from build123d import *

# Parameters (mm, degrees)
SKETCH_1_W        = 50
SKETCH_1_H        = 2
EXTRUDE_1_DEPTH   = 15
EXTRUDE_1_2_DEPTH = 15
SKETCH_2_W        = 50
SKETCH_2_H        = 12.8
EXTRUDE_2_DEPTH   = 2
FILLET_1_R        = 2


with BuildPart() as part:
    # Sketch 1 → Extrude 1 (new body)
    with BuildSketch(Plane.XY):
        with Locations((25, -1)):
            Rectangle(SKETCH_1_W, SKETCH_1_H)
    extrude(amount=EXTRUDE_1_DEPTH)



with BuildPart() as body_2:
    # Sketch 1 → Extrude 1 2 (new body)
    with BuildSketch(Plane.XY):
        with Locations((25, 9.8)):
            Rectangle(SKETCH_1_W, SKETCH_1_H)
    extrude(amount=EXTRUDE_1_2_DEPTH)


with BuildPart() as part_1:
    add(part.part)

    add(body_2.part)  # Extrude 2 merges body 2
    # Sketch 2 → Extrude 2 (add)
    with BuildSketch(Plane.XY.offset(15)):
        with Locations((25, 4.4)):
            Rectangle(SKETCH_2_W, SKETCH_2_H)
    extrude(amount=-EXTRUDE_2_DEPTH)

    # Fillet 1
    fillet_1_edges = [part_1.edges().sort_by_distance(p)[0] for p in [
        (25, 0, 0),
        (25, 8.8, 0),
    ]]
    fillet(fillet_1_edges, radius=FILLET_1_R - 0.0001)  # a hair under: the kernel refuses the full size


solid = part_1.part
Input: part model. Units: mm. Frame: model coordinates. A direction names the side the tool comes from. Give positions to 0.01 mm unless a question says otherwise; leave off trailing zeros. Order: outer loops, then holes, each group sorted by start corner. A loop starts at its lowest first (then second) coordinate and runs counter-clockwise, first axis right, second up. Notation, with made-up numbers: (78, -25.5) - (93, -25.5) arc R30 ccw to (93, 4.5) - close; hole circle Ø4 at (36, 77). An arc over 180 degrees is marked (long way). Answer as a JSON object with one key per item and string values. Group by question number.
Q1. First-contact query: pin 1 Ø2.5 at (x, y) = (37.5, 6.5) entering from -Z. Flat tip, straight axial feed; report the tip coordinate or a pass-through.
Q2. Cut plane C-C, the plane y = 6. Output: boundary loops of the cut face in (x, z).
Q3. Cut plane D-D, the plane y = 9.75. Output: boundary loops of the cut face in (x, z), then the cut area to 3 significant figures.
Q4. Line query: probe 1 along Y at (x, z) = (12, 2.25); probe 2 along Z at (x, y) = (25, 5.5); probe 3 along Y at (x, z) = (21, 1.5). Output: solid intervals per line, ascending.
Q5. Cut plane A-A, the plane z = 6.5. Output: boundary loops of the cut face in (x, y), then the cut area to 3 significant figures.
Q6. Mould query, pull axis Y, two halves, no side actions, for faces 1 (the face through (25, -2, 7)), 2 (the face through (25, 10.8, 7)), 3 (the face through (25, 4, 13)). Classes: pulls with the +Y half, pulls with the -Y half, needs draft (parallel to the pull), parting line crosses it, or undercut.
Q7. Set-up query: faces 4 (the face through (25.35, 9.37, 0.6)), 5 (the face through (25, 4, 15)). Return all of +Z, -Z, +X, -X, +Y, -Y with unobstructed straight access to the full face (end or side cutting, diameter ignored); none if empty.
Results:
{
 "1": {"pin 1": "z = 13"},
 "2": {"outline": "(0, 13) - (50, 13) - (50, 15) - (0, 15) - close"},
 "3": {"outline": "(0, 0.3) - (50, 0.3) - (50, 15) - (0, 15) - close", "area": "735 mm^2"},
 "4": {"probe 1": "-2 to 0, 8.8 to 10.8", "probe 2": "13 to 15", "probe 3": "-2 to -0.06, 8.86 to 10.8"},
 "5": {"outline": "(0, -2) - (50, -2) - (50, 0) - (0, 0) - close; (0, 8.8) - (50, 8.8) - (50, 10.8) - (0, 10.8) - close", "area": "200 mm^2"},
 "6": {"face 1": "pulls with the -Y half", "face 2": "pulls with the +Y half", "face 3": "undercut"},
 "7": {"face 4": "-Z, +X, -X", "face 5": "+Z, +X, -X, +Y, -Y"}
}
